Here's how the part is built. I have some questions about the finished solid (model axes, mm). Face numbers are marked on the shaded views. A direction names the side the tool comes from. Give positions to 0.01 mm unless a question says otherwise; leave off trailing zeros. Loops run counter-clockwise (first coordinate to the right, second up) from the corner with the lowest first, then second, coordinate; pieces in that order, holes last. Notation, with made-up numbers: M 34.5,61 L 46.5,61 A9 cw 46.5,67 Z; hole C 62.5,17 d3. An arc over 180 degrees is marked long. Write item = value, one per line. Start each with the question number.
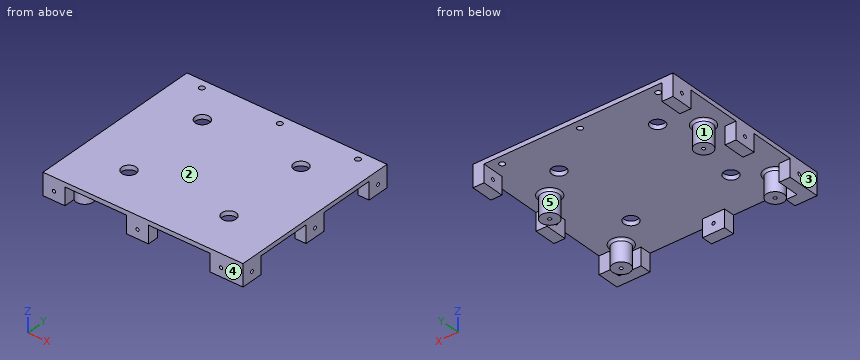
Autodesk Inventor part; units mm, degrees
ref_plane "YZ Plane" through (0, 0, 0) normal (1, 0, 0) x (0, 1, 0)
ref_plane "XZ Plane" through (0, 0, 0) normal (0, 1, 0) x (-1, 0, 0)
ref_plane "XY Plane" through (0, 0, 0) normal (0, 0, 1) x (1, 0, 0)
ref_plane "Work Plane1" through (0, 0, 0) normal (0, 0, 1) x (1, 0, 0)
sketch "Sketch1" plane through (0, 0, 0) normal (0, 0, 1) x (1, 0, 0)
  circle A0 centre (-10, 5) radius 2
  circle A1 centre (-80, 5) radius 2.426
  circle A2 centre (-10, 45) radius 2
  circle A3 centre (-80, 45) radius 2
  circle A4 centre (-10, 5) radius 4
  circle A5 centre (-80, 5) radius 4
  circle A6 centre (-10, 45) radius 4
  circle A7 centre (-80, 45) radius 4
  point P0 (0, 0)
  dimension "d0" = 8
  dimension "d1" = 8
  dimension "d2" = 8
  dimension "d3" = 8
extrude "Extrusion1" add sketch "Sketch1" along normal blind 10 contours A0 | A1 | A2 | A3 | A4 | A5 | A6 | A7
sketch "Sketch2" plane through (-10, 5, 10) normal (0, 0, 1) x (1, 0, 0)
  circle A0 centre (0, 0) radius 4
  circle A1 centre (0, 0) radius 0.75
  circle A2 centre (-70, 0) radius 4
  circle A3 centre (-70, 0) radius 0.75
  circle A4 centre (0, 40) radius 4
  circle A5 centre (0, 40) radius 0.75
  circle A6 centre (-70, 40) radius 4
  circle A7 centre (-70, 40) radius 0.75
  point P0 (10, -5)
  dimension "d6" = 1.5
  dimension "d7" = 1.5
  dimension "d8" = 1.5
  dimension "d9" = 1.5
extrude "Extrusion2" cut sketch "Sketch2" against normal blind 10 contours A1 | A3 | A5 | A7
sketch "Sketch3" plane through (-10, 5, 10) normal (0, 0, 1) x (1, 0, 0)
  line L0 (-75, -10) -> (5, -10)
  line L1 (-80, 45) -> (-80, -5)
  line L2 (5, 50) -> (-75, 50)
  line L3 (10, -5) -> (10, 45)
  line L4 (-80.5, -10.5) -> (10.5, -10.5)
  line L5 (10.5, -10.5) -> (10.5, 70)
  line L6 (10.5, 70) -> (-80.5, 70)
  line L7 (-80.5, 70) -> (-80.5, -10.5)
extrude "Extrusion3" add sketch "Sketch3" along normal blind 2
sketch "Sketch4" plane through (-10, 5, 12) normal (0, 0, 1) x (1, 0, 0)
  line L0 (-80.5, 70) -> (10.5, 70)
  circle A0 centre (-12.25, 9.625) radius 3.25
  circle A1 centre (-57.75, 9.625) radius 3.25
  circle A2 centre (-12.25, 49.875) radius 3.25
  circle A3 centre (-57.75, 50.6331) radius 3.25
  point P0 (10, -5)
  point P1 (10.5, -10.5)
  dimension "d18" = 6.5
  dimension "d19" = 6.5
  dimension "d20" = 6.5
  dimension "d21" = 6.5
extrude "Extrusion4" cut sketch "Sketch4" against normal blind 2
sketch "Sketch5" plane through (0.5, -5.5, 10) normal (1, 0, 0) x (0, 0, -1)
  point P0 (10, 5.5)
sketch "Sketch6" plane through (0.5, -5.5, 10) normal (1, 0, 0) x (0, 0, -1)
  point P0 (10, 5.5)
sketch "Sketch7" plane through (0.5, -5.5, 10) normal (1, 0, 0) x (0, 0, -1)
  line L0 (0, 0) -> (0, 80.5)
  line L1 (0, 0) -> (8, 0)
  line L2 (8, 0) -> (8, 10)
  line L3 (8, 10) -> (0, 10)
  line L4 (0, 10) -> (0, 0)
  circle A0 centre (4, 5) radius 0.75
  point P0 (10, 5.5)
  dimension "d24" = 8
  dimension "d25" = 10
  dimension "d26" = 1.5
extrude "Extrusion5" add sketch "Sketch7" against normal blind 5
sketch "Sketch8" plane through (-90.5, -5.5, 12) normal (0, -1, 0) x (1, 0, 0)
  line L0 (86, -10) -> (86, -2)
  line L1 (86, -10) -> (76, -10)
  line L2 (76, -10) -> (76, -2)
  line L3 (76, -2) -> (86, -2)
  line L4 (86, -2) -> (86, -10)
  circle A0 centre (81, -6) radius 0.75
  point P0 (90.5, -12)
  dimension "d29" = 10
  dimension "d30" = 8
  dimension "d31" = 1.5
extrude "Extrusion6" add sketch "Sketch8" against normal blind 5
fillet "Fillet1" radius 1 1 edges at (-14, 5, 10)
sketch "Sketch9" plane through (-90.5, -5.5, 12) normal (0, -1, 0) x (1, 0, 0)
  line L0 (0, -2) -> (76, -2)
  line L1 (0, -2) -> (10, -2)
  line L2 (10, -2) -> (10, -10)
  line L3 (10, -10) -> (0, -10)
  line L4 (0, -10) -> (0, -2)
  circle A0 centre (5, -6) radius 0.75
  point P0 (90.5, -12)
  dimension "d35" = 10
  dimension "d36" = 8
  dimension "d37" = 1.5
extrude "Extrusion7" add sketch "Sketch9" against normal blind 5
sketch "Sketch10" plane through (-90.5, -5.5, 12) normal (-1, 0, 0) x (0, 0, 1)
  line L0 (-2, 5) -> (-2, 0)
  line L1 (-2, 5) -> (-10, 5)
  line L2 (-10, 5) -> (-10, 15)
  line L3 (-10, 15) -> (-2, 15)
  line L4 (-2, 15) -> (-2, 5)
  circle A0 centre (-6, 10) radius 0.75
  point P0 (-12, 5.5)
  point P1 (-2, 10)
  point P2 (-10, 10)
  dimension "d40" = 8
  dimension "d41" = 10
  dimension "d42" = 1.5
extrude "Extrusion8" add sketch "Sketch10" against normal blind 5
fillet "Fillet2" radius 1 1 edges at (-84, 5, 10)
sketch "Sketch11" plane through (-90.5, -5.5, 12) normal (0, -1, 0) x (1, 0, 0)
  line L0 (10, -2) -> (76, -2)
  line L1 (76, -2) -> (10, -2)
  circle A0 centre (43, -6) radius 0.75
  line L2 (43, -2) -> (38, -2)
  line L3 (38, -2) -> (38, -10)
  line L4 (38, -10) -> (48, -10)
  line L5 (48, -10) -> (48, -2)
  point P0 (90.5, -12)
  dimension "d47" = 1.5
  dimension "d48" = 5
  dimension "d49" = 8
  dimension "d50" = 10
extrude "Extrusion9" add sketch "Sketch11" against normal blind 5
sketch "Sketch12" plane through (-90.5, -5.5, 12) normal (-1, 0, 0) x (0, 0, 1)
  point P0 (-12, 5.5)
fillet "Fillet3" radius 1 2 edges at (-84, 45, 10) (-14, 45, 10)
sketch "Sketch13" plane through (-90.5, -5.5, 12) normal (-1, 0, 0) x (0, 0, 1)
  line L0 (-10, 0) -> (0, 0)
  line L1 (0, 0) -> (0, 80.5)
  circle A0 centre (-6, 40.25) radius 0.75
  line L2 (-10, 40.25) -> (-10, 45.25)
  line L3 (-10, 45.25) -> (-2, 45.25)
  line L4 (-2, 45.25) -> (-2, 35.25)
  line L5 (-2, 80.5) -> (-2, 15)
  line L6 (-2, 35.25) -> (-10, 35.25)
  line L7 (-10, 35.25) -> (-10, 40.25)
  point P0 (-12, 5.5)
  dimension "d56" = 1.5
  dimension "d57" = 5
  dimension "d58" = 8
  dimension "d59" = 10
  dimension "d60" = 8
extrude "Extrusion10" add sketch "Sketch13" against normal blind 5
sketch "Sketch14" plane through (0.5, -5.5, 12) normal (1, 0, 0) x (0, 0, -1)
  line L0 (10, 35.25) -> (10, 45.25)
  circle A0 centre (6, 40.25) radius 0.75
  circle A1 centre (6, 40.25) radius 0.75
  line L1 (10, 40.25) -> (10, 35.25)
  line L2 (10, 35.25) -> (2, 35.25)
  line L3 (2, 10) -> (2, 80.5)
  line L4 (2, 35.25) -> (2, 45.25)
  line L5 (2, 45.25) -> (10, 45.25)
  line L6 (10, 45.25) -> (10, 40.25)
  point P0 (12, 5.5)
  dimension "d63" = 1.5
  dimension "d65" = 8
  dimension "d66" = 10
  dimension "d67" = 8
extrude "Extrusion11" add sketch "Sketch14" against normal blind 5
sketch "Sketch15" plane through (0.5, -5.5, 12) normal (1, 0, 0) x (0, 0, -1)
  line L0 (2, 80.5) -> (0, 80.5)
  line L1 (2, 80.5) -> (10, 80.5)
  line L2 (10, 80.5) -> (10, 70.5)
  line L3 (10, 70.5) -> (2, 70.5)
  line L4 (2, 70.5) -> (2, 80.5)
  circle A0 centre (6, 75.5) radius 0.75
  point P0 (12, 5.5)
  dimension "d70" = 8
  dimension "d71" = 10
  dimension "d73" = 1.5
extrude "Extrusion12" add sketch "Sketch15" against normal blind 5
sketch "Sketch16" plane through (-90.5, -5.5, 12) normal (-1, 0, 0) x (0, 0, 1)
  line L0 (-2, 80.5) -> (0, 80.5)
  line L1 (-10, 70.5) -> (-2, 70.5)
  line L2 (-2, 80.5) -> (-10, 80.5)
  line L3 (-10, 80.5) -> (-10, 70.5)
  line L4 (-10, 70.5) -> (-2, 70.5)
  line L5 (-2, 70.5) -> (-2, 80.5)
  circle A0 centre (-6, 75.5) radius 0.75
  circle A1 centre (-6, 75.5) radius 0.75
  point P0 (-12, 5.5)
extrude "Extrusion13" add sketch "Sketch16" against normal blind 5
sketch "Sketch17" plane through (-10, 5, 10) normal (0, 0, -1) x (-1, 0, 0)
  circle A0 centre (35, 66) radius 1.25
  circle A1 centre (70.5, 66) radius 1.25
  circle A2 centre (-0.5, 66) radius 1.25
  point P0 (-10, -5)
  point P1 (75.5, 70)
  dimension "d79" = 2.5
  dimension "d83" = 2.5
  dimension "d85" = 2.5
extrude "Extrusion14" cut sketch "Sketch17" against normal blind 2
sketch "Sketch18" plane through (-10, 5, 12) normal (0, 0, 1) x (1, 0, 0)
  point P0 (10, -5)
properties part number "Down" material "Nylon, molybdenum disulphide"
Q1. If I drill on line 1 along Y through (x, z) = (-1.1, 6); line 2 along Y through (x, z) = (-67.75, 10.6) (3 decimals); line 3 along Z through (x, y) = (-47.5, -4.05), over which ranges is the centre line in solid material (lowest first)?
Q2. If we section it at B-B, the plane z = 3.5: State how many separate pieces and enclosed holes the cut face has, then the cut area to 3 significant figures.
Q3. If we section it at A-A, the plane x = -45: List the corners of the cut face in (y, z) for me.
Q4. Will these pins go through, and if not, where does the flat tip stop? pin 1 (1.5 mm diameter, centred on x = -88.5, y = 35.5, fed in from -Z); pin 2 (11 mm diameter, centred on x = -6, y = -3, fed in from -Z); pin 3 (2.5 mm diameter, centred on x = -84, z = 5.5, fed in from +Y); pin 4 (1.2 mm diameter, centred on x = -80, y = 45, fed in from -Z).
Q5. If we section it at C-C, the plane y = 53.5: List the corners of the cut face in (x, z) for me.
Q6. If we section it at D-D, the plane y = 66.5: List the corners of the cut face in (x, z) for me, then the cut area to 3 significant figures.
Q7. We'd pull the mould along X, two halves only. Please class the marked faces 3, 4 and 5: pulls with the +X half, pulls with the -X half, needs draft (parallel to the pull), parting line crosses it, or undercut.
Q8. On a 3-axis mill with a long thin cutter (end or side, diameter ignored), from which of +Z, -Z, +X, -X, +Y, -Y can I reach the whole of each face in a straight line? I mean the marked faces 1 and 2. Say none if no direction works.
Resolved:
q1.line_1 = -5.5 to -1.25, 0.25 to 4.5, 29.75 to 34, 35.5 to 39.75, 65 to 69.25, 70.75 to 75
q1.line_2 = -5.5 to 11.375, 17.875 to 52.383, 58.883 to 75
q1.line_3 = 2 to 5.25, 6.75 to 12
q2.separate_pieces = 11
q2.enclosed_holes = 4
q2.area = 644 mm²
q3.outline = M -5.5,2 L -0.5,2 L -0.5,10 L 69.75,10 L 69.75,12 L -5.5,12 Z; M 72.25,10 L 75,10 L 75,12 L 72.25,12 Z
q4.pin_1 = 2
q4.pin_2 = 0
q4.pin_3 = 47.9
q4.pin_4 = 10
q5.outline = M -90.5,10 L -70.2,10 L -70.2,12 L -90.5,12 Z; M -65.3,10 L -25.19,10 L -25.19,12 L -65.3,12 Z; M -19.31,10 L 0.5,10 L 0.5,12 L -19.31,12 Z
q6.outline = M -90.5,2 L -85.5,2 L -85.5,10 L -4.5,10 L -4.5,2 L 0.5,2 L 0.5,12 L -90.5,12 Z
q6.area = 262 mm²
q7.face_3 = pulls with the -X half
q7.face_4 = needs draft
q7.face_5 = undercut
q8.face_1 = -Z
q8.face_2 = +Z, +X, -X, +Y, -Y
